Can you work these out from the model? Positions are in its coordinate system, mm. A direction names the side the tool comes from. Coordinates: 2 decimals unless noted, no trailing zeros. Write each loop counter-clockwise with the first axis right and the second up, starting at its lowest first coordinate (ties: lowest second). Pieces come first, ordered by that corner, then holes. Notation, with made-up numbers: (-16, 28.5) -> (41, 28.5) arc R25 ccw to (41, 62.5) -> close; hole circle Ø7 at (59, 37). An arc over 180 degrees is marked (long way). Use one line per item in the form item = value.
```python
from build123d import *

# Parameters (mm, degrees)
BOSS_EXTRUDE1_DEPTH = 31.72


with BuildPart() as part:
    # Sketch1 → Boss-Extrude1 (new body)
    with BuildSketch(Plane.XY):
        with BuildLine():
            Line((-0.9, 2.116601049), (-0.9, 0.9))
            Line((-0.9, 0.9), (-2.116601049, 0.9))
            ThreePointArc((-2.116601049, 0.9), (-2.3, 0), (-2.116601049, -0.9))
            Line((-2.116601049, -0.9), (-0.9, -0.9))
            Line((-0.9, -0.9), (-0.9, -2.116601049))
            ThreePointArc((-0.9, -2.116601049), (0, -2.3), (0.9, -2.116601049))
            Line((0.9, -2.116601049), (0.9, -0.9))
            Line((0.9, -0.9), (2.116601049, -0.9))
            ThreePointArc((2.116601049, -0.9), (2.3, 0), (2.116601049, 0.9))
            Line((2.116601049, 0.9), (0.9, 0.9))
            Line((0.9, 0.9), (0.9, 2.116601049))
            ThreePointArc((0.9, 2.116601049), (0, 2.3), (-0.9, 2.116601049))
        make_face()
    extrude(amount=BOSS_EXTRUDE1_DEPTH)

    # Sketch2 → Cut-Revolve3 (revolve, cut)
    with BuildSketch(Plane(origin=(0, 0, 0), x_dir=(1, 0, 0), z_dir=(0, 1, 0)), mode=Mode.PRIVATE) as cut_revolve3_sk:
        Polygon((0.228583367, 0.219399408), (2.871914227, 0.219399408), (2.871914227, -0.728161621), align=None)
        Polygon((2.871914227, -30.991838379), (0.228583367, -31.939399408), (2.871914227, -31.939399408), align=None)
    revolve(cut_revolve3_sk.sketch.rotate(Axis((0, 0, -10.126702137), (0, 0, 1)), 156.964321077), axis=Axis((0, 0, -10.126702137), (0, 0, 1)), mode=Mode.SUBTRACT)


solid = part.part
```
Q1. Will these pins go through, and if not, where does the flat tip stop? pin 1 (1.3 mm diameter, centred on x = 1.5, z = 16.5, fed in from -Y); pin 2 (1 mm diameter, centred on y = 1.5, z = 18.5, fed in from +X); pin 3 (0.6 mm diameter, centred on y = -1.5, z = 18.5, fed in from -X).
Return value:
pin_1 = -2.14
pin_2 = 0.9
pin_3 = -0.9
Q2. If I drill on line 1 (X direction, y = -1.7, z = 22); line 2 (Z direction, x = -0.45, y = 1.1), over which ranges is the centre line in solid material (lowest first)? Write a range as from..to.
Return value:
line_1 = -0.9..0.9
line_2 = 0.12..31.6
Q3. For faces 1 (the flat face through (1.5, 0.9, 15.6)), 2 (the flat face through (-0.9, 1.5, 15.6)), 3 (the flat face through (-1.5, -0.9, 15.6)), 4 (the flat face through (1.5, -0.9, 15.6)), which set-ups out of +Z, -Z, +X, -X, +Y, -Y let a thin tool reach every point of the face, with its end or its side?
Return value:
face_1 = +Z, -Z, +X, +Y
face_2 = +Z, -Z, -X, +Y
face_3 = +Z, -Z, -X, -Y
face_4 = +Z, -Z, +X, -Y
Q4. Suppose I cut it at A-A (z = 15). Write out the boundary of the cut face in (x, y), then the cut area to 3 significant figures.
Return value:
outline = (-2.12, -0.9) -> (-0.9, -0.9) -> (-0.9, -2.12) arc R2.3 ccw to (0.9, -2.12) -> (0.9, -0.9) -> (2.12, -0.9) arc R2.3 ccw to (2.12, 0.9) -> (0.9, 0.9) -> (0.9, 2.12) arc R2.3 ccw to (-0.9, 2.12) -> (-0.9, 0.9) -> (-2.12, 0.9) arc R2.3 ccw to start
area = 12.9 mm2
